from build123d import *

# Parameters (mm, degrees)
F0_W     = 300
F0_H     = 300
F1_DEPTH = 25
F3_T     = -10
F4_DEPTH = 4
F5_W     = 300
F5_H     = 300
F5_W_2   = 292
F5_H_2   = 292
F6_DEPTH = 4


with BuildPart() as f1:
    # F0 (on Top) → F1 (new body)
    with BuildSketch(Plane.XY):
        with Locations((95.5334320664, 89.3530972302)):
            Rectangle(F0_W, F0_H)
    extrude(amount=F1_DEPTH)

    # F3
    f3_openings = [f1.faces().sort_by_distance(p)[0] for p in [
        (95.533432, 89.353097, 25),
    ]]
    offset(amount=F3_T, openings=f3_openings)

    # F2 (on face) → F4 (cut)
    with BuildSketch(Plane.XZ.offset(60.6469027698)):
        with BuildLine():
            ThreePointArc((-36.1368541132, 0), (-35.4589387768, 1.4324265188), (-35.2262808864, 2.9999995604))
            ThreePointArc((-35.2262808864, 2.9999995604), (-42.1910810125, 8.1645687544), (-45.1101618284, 0))
            Line((-45.1101618284, 0), (-36.1368541132, 0))
        make_face()
    extrude(amount=-F4_DEPTH, mode=Mode.SUBTRACT)

    # F5 (on face) → F6 (join)
    with BuildSketch(Plane.XY.offset(25)):
        with Locations((95.5334320664, 89.3530972302)):
            Rectangle(F5_W, F5_H)
        with Locations((95.5334320664, 89.3530972302)):
            Rectangle(F5_W_2, F5_H_2, mode=Mode.SUBTRACT)
    extrude(amount=F6_DEPTH)


solid = f1.part
Work out the finished part from the listing and answer in its coordinate system (mm). A direction names the side the tool comes from. Give positions to 0.01 mm unless a question says otherwise; leave off trailing zeros. Order: outer loops, then holes, each group sorted by start corner. A loop starts at its lowest first (then second) coordinate and runs counter-clockwise, first axis right, second up. Notation, with made-up numbers: (25.25, 23.25) - (39.25, 23.25) arc R18 ccw to (39.25, 49.25) - close; hole circle Ø1 at (-7.75, 4.5). An arc over 180 degrees is marked (long way). Answer as CSV lines item,"result". Start each with the question number.
Q1. The part is cut by section C-C (y = -7). Write down the section's boundary in (x, z).
Q2. Given pin 1 Ø6.5 at (x, z) = (-40, 5) entering from -Y; pin 2 Ø10 at (x, y) = (111.5, 103) entering from +Z, each flat-ended and moving along its own axis, determine where each tip first touches the part or whether it passes through.
Q3. The part is cut by section B-B (x = 121.5). Write down the section's boundary in (y, z).
Q4. Find the intervals of material crossed by L1, parallel to X at y = -58.9, z = 3; L2, parallel to Y at x = 223, z = 24; L3, parallel to X at y = 109.5, z = 14.5, in increasing order. Write a range as [from, to].
Q5. For faces 1 (the face through (-54.467, 87, 14)), 2 (the face through (-41, -56.647, 4)), 3 (the face through (-44.467, 87, 17)), determine the directions among +Z, -Z, +X, -X, +Y, -Y from which every point of the face is accessible in a straight line to the end or side of a thin tool.
Q6. The part is cut by section A-A (z = 19.75). Write down the section's boundary in (x, y), then the cut area to 3 significant figures.
Check result:
1,outline,"(-54.47, 0) - (245.53, 0) - (245.53, 29) - (241.53, 29) - (241.53, 25) - (235.53, 25) - (235.53, 10) - (-44.47, 10) - (-44.47, 25) - (-50.47, 25) - (-50.47, 29) - (-54.47, 29) - close"
2,pin 1,"stops at y = -56.65"
2,pin 2,"stops at z = 10"
3,outline,"(-60.65, 0) - (239.35, 0) - (239.35, 29) - (235.35, 29) - (235.35, 25) - (229.35, 25) - (229.35, 10) - (-50.65, 10) - (-50.65, 25) - (-56.65, 25) - (-56.65, 29) - (-60.65, 29) - close"
4,L1,"x = [-54.47, -46.02], [-35.23, 245.53]"
4,L2,"y = [-60.65, -50.65], [229.35, 239.35]"
4,L3,"x = [-54.47, -44.47], [235.53, 245.53]"
5,face 1,"+Z, -Z, -X, +Y, -Y"
5,face 2,"-Y"
5,face 3,"+Z"
6,outline,"(-54.47, -60.65) - (245.53, -60.65) - (245.53, 239.35) - (-54.47, 239.35) - close; hole (-44.47, -50.65) - (235.53, -50.65) - (235.53, 229.35) - (-44.47, 229.35) - close"
6,area,"11,600 mm²"
